Verification items for the finished model (mm, model axes). Face numbers are marked on the shaded views. Give positions to 0.01 mm unless a question says otherwise; leave off trailing zeros. Loops run counter-clockwise (first coordinate to the right, second up) from the corner with the lowest first, then second, coordinate; pieces in that order, holes last. Notation, with made-up numbers: M 79,34 L 98,34 A26 cw 98,68 Z; hole C 1.5,62 d2. An arc over 180 degrees is marked long. Use CSV: the item, a comma, the result in double quotes.
from build123d import *

# Parameters (mm, degrees)
BOSS_EXTRUDE1_DEPTH = 3
SKETCH2_W           = 12.2
SKETCH2_H           = 23
CUT_EXTRUDE1_DEPTH  = 4
SKETCH5_R           = 3.925
SKETCH5_R_2         = 0.75
CUT_EXTRUDE2_DEPTH  = 3


with BuildPart() as part:
    # Sketch1 → Boss-Extrude1 (new body)
    with BuildSketch(Plane.XY):
        with BuildLine():
            Line((-29.761795946, -16.735008518), (-29.761795946, -27.401277683))
            Line((-29.761795946, -27.401277683), (-24.065046346, -27.401277683))
            Line((-24.065046346, -27.401277683), (-24.065046346, -40.380088331))
            Line((-24.065046346, -40.380088331), (-26.761795946, -40.380088331))
            Line((-26.761795946, -40.380088331), (-30.96655582, -40.372207157))
            Line((-30.96655582, -40.372207157), (-30.96655582, -46.377768313))
            Line((-30.96655582, -46.377768313), (-27.761795946, -46.377768313))
            Line((-27.761795946, -46.377768313), (-2.624484573, -46.377768313))
            ThreePointArc((-2.624484573, -46.377768313), (-1.210271011, -45.791981876), (-0.624484573, -44.377768313))
            Line((-0.624484573, -44.377768313), (-0.624484573, -3.377768313))
            ThreePointArc((-0.624484573, -3.377768313), (-1.210271011, -1.963554751), (-2.624484573, -1.377768313))
            Line((-2.624484573, -1.377768313), (-26.540138154, -1.377768313))
            Line((-26.540138154, -1.377768313), (-26.540138154, -6.377768313))
            Line((-26.540138154, -6.377768313), (-29.540138154, -6.377768313))
            Line((-29.540138154, -6.377768313), (-29.540138154, -1.377768313))
            Line((-29.540138154, -1.377768313), (-34.506351605, -1.377768313))
            Line((-34.506351605, -1.377768313), (-34.506351605, -11.735008518))
            Line((-34.506351605, -11.735008518), (-29.761795946, -11.735008518))
            Line((-29.761795946, -11.735008518), (-24.065046346, -11.735008518))
            Line((-24.065046346, -11.735008518), (-24.065046346, -16.735008518))
            Line((-24.065046346, -16.735008518), (-29.761795946, -16.735008518))
        make_face()
    extrude(amount=BOSS_EXTRUDE1_DEPTH)

    # Sketch2 → Cut-Extrude1 (cut, through all)
    with BuildSketch(Plane.XY.offset(3)):
        with Locations((-10.143120504, -28.115803741)):
            Rectangle(SKETCH2_W, SKETCH2_H)
    extrude(amount=-CUT_EXTRUDE1_DEPTH, mode=Mode.SUBTRACT)

    # Sketch5 → Cut-Extrude2 (cut)
    with BuildSketch(Plane.XY.offset(3)):
        with Locations((-10.143120504, -16.615803741)):
            Circle(SKETCH5_R)
        with Locations((-10.143120504, -41.615803741)):
            Circle(SKETCH5_R_2)
    extrude(amount=-CUT_EXTRUDE2_DEPTH, mode=Mode.SUBTRACT)


solid = part.part
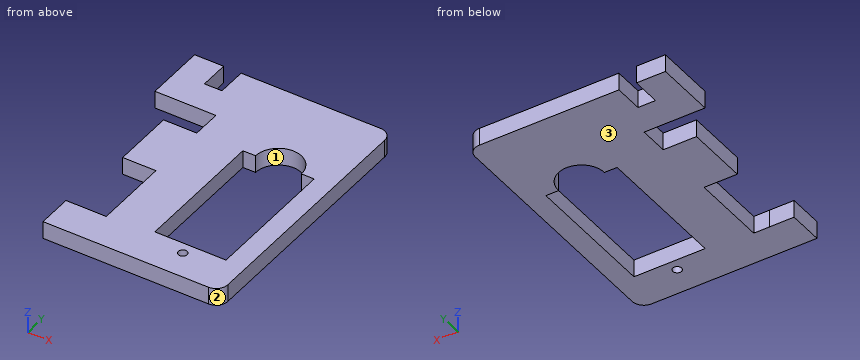
(1) Section check C-C on z = 2.3. Record the cut outline in (x, y) (3 decimals), plus the area to 3 significant figures.
Calculated:
outline,"M -34.506,-11.735 L -24.065,-11.735 L -24.065,-16.735 L -29.762,-16.735 L -29.762,-27.401 L -24.065,-27.401 L -24.065,-40.38 L -26.762,-40.38 L -30.967,-40.372 L -30.967,-46.378 L -2.624,-46.378 A2 ccw -0.624,-44.378 L -0.624,-3.378 A2 ccw -2.624,-1.378 L -26.54,-1.378 L -26.54,-6.378 L -29.54,-6.378 L -29.54,-1.378 L -34.506,-1.378 Z; hole M -16.243,-39.616 L -4.043,-39.616 L -4.043,-16.616 L -6.218,-16.616 A3.925 ccw -14.068,-16.616 L -16.243,-16.616 Z; hole C -10.143,-41.616 d1.5"
area,"942 mm²"
(2) Mould release check, pull along X, two halves, no side actions. Record for the marked faces 1, 2 and 3: released by +X, released by -X, zero draft, split by the parting line, or undercut.
Calculated:
face 1,"undercut"
face 2,"released by +X"
face 3,"zero draft"
(3) Depth check by flat-ended pin: pin 1 Ø1.5 at (y, z) = (-23, 2.5) entering from -X; pin 2 Ø1.5 at (y, z) = (-43.5, 2) entering from -X. Enter the tip coordinate at first touch or a pass-through.
Calculated:
pin 1,"stops at x = -29.76"
pin 2,"stops at x = -30.97"
(4) Section check D-D on x = -31.5. Record the cut outline in (y, z) (3 decimals), plus the area to 3 significant figures.
Calculated:
outline,"M -11.735,0 L -1.378,0 L -1.378,3 L -11.735,3 Z"
area,"31.1 mm²"
(5) Section check B-B on x = -7. Record the cut outline in (y, z).
Calculated:
outline,"M -46.38,0 L -39.62,0 L -39.62,3 L -46.38,3 Z; M -14.26,0 L -1.38,0 L -1.38,3 L -14.26,3 Z"
(6) Scan lines: L1, parallel to Y at x = -25.5, z = 1.65 (3 decimals); L2, parallel to Y at x = -29, z = 0.3 (3 decimals); L3, parallel to X at y = -32, z = 0.85. Record each from-to range of solid material in increasing order. Write a range as from..to.
Calculated:
L1,"y = -46.378..-40.38, -27.401..-16.735, -11.735..-1.378"
L2,"y = -46.378..-40.376, -27.401..-16.735, -11.735..-6.378"
L3,"x = -24.07..-16.24, -4.04..-0.62"
(7) Section check A-A on y = -18. Record the cut outline in (x, z).
Calculated:
outline,"M -29.76,0 L -16.24,0 L -16.24,3 L -29.76,3 Z; M -4.04,0 L -0.62,0 L -0.62,3 L -4.04,3 Z"
